Answer from the drawing. Dimensions are ordinates in mm from the lowest x, y and z of the part. A direction names the side the tool comes from. Give positions to 0.01 mm unless a question says otherwise; leave off trailing zeros. Loops run counter-clockwise (first coordinate to the right, second up) from the corner with the lowest first, then second, coordinate; pieces in that order, holes last.
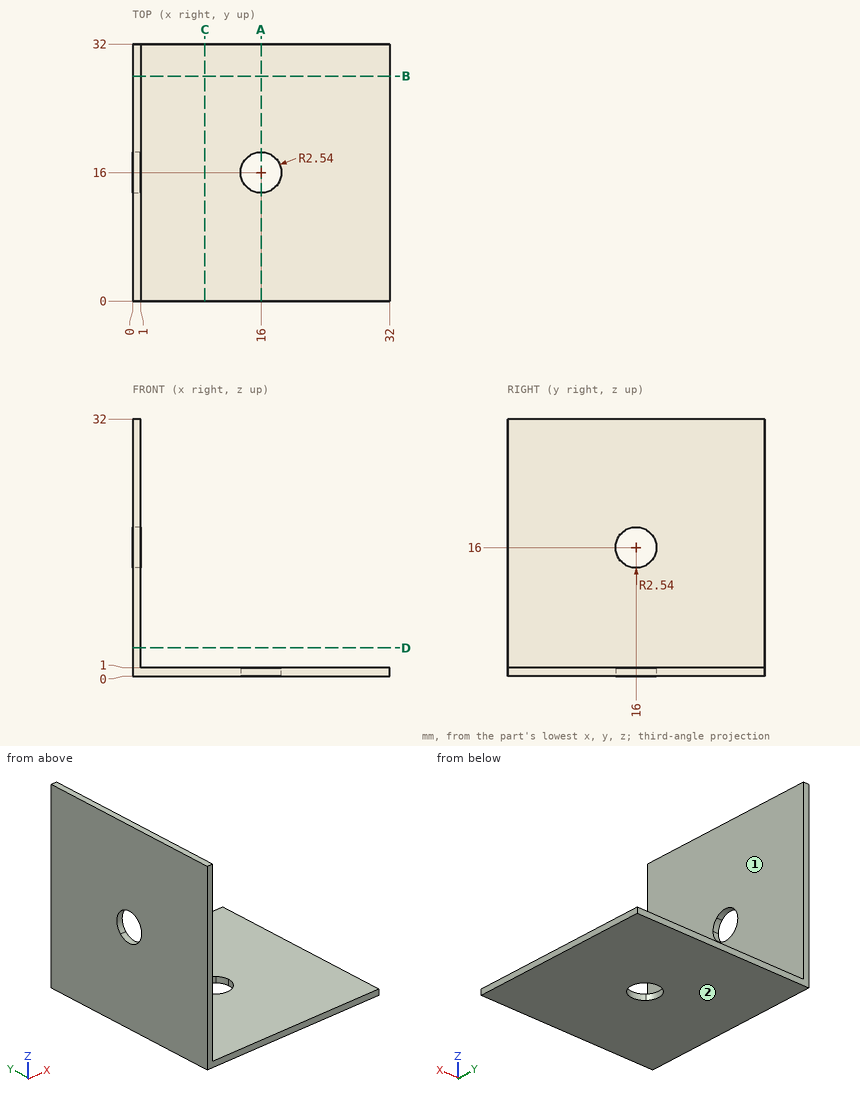
Item 1: Find section B-B, the plane y = 28. Write down the section's boundary in (x, z), plus the area to 3 significant figures.
Item 2: Find section D-D, the plane z = 3.5. Write down the section's boundary in (x, y), plus the area to 3 significant figures.
Item 3: Find section A-A, the plane x = 16. Write down the section's boundary in (y, z).
Item 4: Consider line 1 (X direction, y = 25, z = 11). Determine where the line is inside the solid, lowest interval first.
Item 5: For the marked faces 1 and 2, determine the directions among +Z, -Z, +X, -X, +Y, -Y from which every point of the face is accessible in a straight line to the end or side of a thin tool.
Item 6: Flat-ended cylindrical pins translate along their axes: pin 1 Ø1.5 at (y, z) = (12.5, 18) entering from +X; pin 2 Ø1.5 at (x, y) = (22, 25) entering from +Z. Find the tip coordinate at first contact, or state that the pin passes through.
Item 7: Find section C-C, the plane x = 9. Write down the section's boundary in (y, z), plus the area to 3 significant figures.
Ans:
1. outline: (0, 0) - (32, 0) - (32, 1) - (1, 1) - (1, 32) - (0, 32) - close
1. area: 63.0 mm2
2. outline: (0, 0) - (1, 0) - (1, 32) - (0, 32) - close
2. area: 32.0 mm2
3. outline: (0, 0) - (13.46, 0) - (13.46, 1) - (0, 1) - close; (18.54, 0) - (32, 0) - (32, 1) - (18.54, 1) - close
4. line 1: x = 0 to 1
5. face 1: +Z, +X, +Y, -Y
5. face 2: -Z, +X, -X, +Y, -Y
6. pin 1: stops at x = 1
6. pin 2: stops at z = 1
7. outline: (0, 0) - (32, 0) - (32, 1) - (0, 1) - close
7. area: 32.0 mm2
